```python
from build123d import *

# Parameters (mm, degrees)
SKETCH1_W           = 3
SKETCH1_H           = 8
BOSS_EXTRUDE1_DEPTH = 1.5


with BuildPart() as part:
    # Sketch1 → Boss-Extrude1 (new, symmetric)
    with BuildSketch(Plane.XY):
        Polygon((30.4, -9), (30.4, -5.5), (15.4, -5.5), (15.4, -1.5), (16.4, -1.5), (16.4, 1), (15.4, 1), (15.4, 3.7), (12.4, 3.7), (12.4, 1), (11.4, 1), (11.4, -1.5), (12.4, -1.5), (12.4, -5.5), (-17.4, -5.5), (-17.4, -9), (-24.6, -9), (-24.6, 9.5), (-11.1, 9.5), (-11.1, 12.5), (-6.1, 12.5), (-6.1, 9.5), (0, 9.5), (0, 5.5), (-1, 5.5), (-1, 3), (0, 3), (0, 0.3), (3, 0.3), (3, 3), (4, 3), (4, 5.5), (3, 5.5), (3, 9.5), (27.4, 9.5), (27.4, 12.5), (35.4, 12.5), (35.4, -9), align=None)
        with Locations((25.4, 2)):
            Rectangle(SKETCH1_W, SKETCH1_H, mode=Mode.SUBTRACT)
        with Locations((-7.6, 2)):
            Rectangle(SKETCH1_W, SKETCH1_H, mode=Mode.SUBTRACT)
    extrude(amount=BOSS_EXTRUDE1_DEPTH, both=True)


solid = part.part
```
Geometry: final body of the model. Coordinates: model frame, mm. A direction names the side the tool comes from. Coordinates: 2 decimals unless noted, no trailing zeros. Order: outer loops, then holes, each group sorted by start corner. A loop starts at its lowest first (then second) coordinate and runs counter-clockwise, first axis right, second up. Notation, with made-up numbers: (-26.5, 61) -> (2.5, 61) arc R16 cw to (2.5, 78) -> close; hole circle Ø5 at (-39, 87.5). An arc over 180 degrees is marked (long way). Write each question's results on one line, items separated by ' | '. Start each with the question number.
1) Cut plane A-A, the plane x = -7. Output: boundary loops of the cut face in (y, z).
2) First-contact query: pin 1 (1.5 mm diameter, centred on x = -17.5, z = -0.5, fed in from +Y). Flat tip, straight axial feed; report the tip coordinate or a pass-through.
3) Set-up query: faces 1 (the flat face through (-6.1, 11, 0)), 2 (the flat face through (-11.1, 11, 0)), 3 (the flat face through (-17.4, -7, 0)), 4 (the flat face through (25, -2, 0)). Return all of +Z, -Z, +X, -X, +Y, -Y with unobstructed straight access to the full face (end or side cutting, diameter ignored); none if empty.
4) Cut plane C-C, the plane y = -3.75. Output: boundary loops of the cut face in (x, z), and give its area (3 significant figures).
5) Mould query, pull axis Y, two halves, no side actions, for faces 5 (the flat face through (12, 1, 0)), 6 (the flat face through (23, -5.5, 0)), 7 (the flat face through (6, 2, 1.5)), 8 (the flat face through (31, 12.5, 0)). Classes: released by +Y, released by -Y, zero draft, split by the parting line, or undercut.
6) Cut plane D-D, the plane y = -0.25. Output: boundary loops of the cut face in (x, z).
7) Material intervals for line 1 along X through (y, z) = (3.25, -0.65); line 2 along X through (y, z) = (-0.5, 1.35); line 3 along X through (y, z) = (4.25, -1.3), sorted ascending.
8) Cut plane B-B, the plane y = 2. Output: boundary loops of the cut face in (x, z), and give its area (3 significant figures).
Checks:
1) outline: (-5.5, -1.5) -> (-2, -1.5) -> (-2, 1.5) -> (-5.5, 1.5) -> close; (6, -1.5) -> (12.5, -1.5) -> (12.5, 1.5) -> (6, 1.5) -> close
2) pin 1: y = 9.5
3) face 1: +Z, -Z, +Y | face 2: +Z, -Z, -X, +Y | face 3: +Z, -Z, -Y | face 4: +Z, -Z
4) outline: (-24.6, -1.5) -> (12.4, -1.5) -> (12.4, 1.5) -> (-24.6, 1.5) -> close; (15.4, -1.5) -> (35.4, -1.5) -> (35.4, 1.5) -> (15.4, 1.5) -> close | area: 171 mm^2
5) face 5: undercut | face 6: released by -Y | face 7: zero draft | face 8: released by +Y
6) outline: (-24.6, -1.5) -> (-9.1, -1.5) -> (-9.1, 1.5) -> (-24.6, 1.5) -> close; (-6.1, -1.5) -> (11.4, -1.5) -> (11.4, 1.5) -> (-6.1, 1.5) -> close; (16.4, -1.5) -> (23.9, -1.5) -> (23.9, 1.5) -> (16.4, 1.5) -> close; (26.9, -1.5) -> (35.4, -1.5) -> (35.4, 1.5) -> (26.9, 1.5) -> close
7) line 1: -24.6 to -9.1, -6.1 to -1, 4 to 12.4, 15.4 to 23.9, 26.9 to 35.4 | line 2: -24.6 to -9.1, -6.1 to 11.4, 16.4 to 23.9, 26.9 to 35.4 | line 3: -24.6 to -9.1, -6.1 to -1, 4 to 23.9, 26.9 to 35.4
8) outline: (-24.6, -1.5) -> (-9.1, -1.5) -> (-9.1, 1.5) -> (-24.6, 1.5) -> close; (-6.1, -1.5) -> (0, -1.5) -> (0, 1.5) -> (-6.1, 1.5) -> close; (3, -1.5) -> (12.4, -1.5) -> (12.4, 1.5) -> (3, 1.5) -> close; (15.4, -1.5) -> (23.9, -1.5) -> (23.9, 1.5) -> (15.4, 1.5) -> close; (26.9, -1.5) -> (35.4, -1.5) -> (35.4, 1.5) -> (26.9, 1.5) -> close | area: 144 mm^2
